from build123d import *

# Parameters (mm, degrees)
SKETCH1_W              = 121.666
SKETCH1_H              = 44.958
EXTRUDE1_DEPTH         = 152.4
SKETCH2_W              = 3.683
SKETCH2_H              = 43.292875233
EXTRUDE2_DEPTH         = 152.4
FILLET1_R              = 0.508
LPATTERN1_COUNT        = 23
LPATTERN1_PITCH        = 5.22224
FILLET1_OF_LPATTERN1_R = 0.508
SKETCH4_R              = 1.5875
EXTRUDE3_DEPTH         = 3.81
SKETCH5_R              = 1.5875
EXTRUDE4_DEPTH         = 3.81
SKETCH6_R              = 1.778
EXTRUDE5_DEPTH         = 3.81


with BuildPart() as part:
    # Sketch1 → Extrude1 (new body)
    with BuildSketch(Plane.XY):
        with Locations((60.833, 22.479)):
            Rectangle(SKETCH1_W, SKETCH1_H)
    extrude(amount=-EXTRUDE1_DEPTH)

    # Sketch2 → Extrude2 (cut)
    with BuildSketch(Plane.XY):
        with Locations((3.3655, 25.964437616)):
            Rectangle(SKETCH2_W, SKETCH2_H)
    extrude2 = extrude(amount=-EXTRUDE2_DEPTH, mode=Mode.SUBTRACT)

    # Fillet1
    fillet1_edges = [part.edges().sort_by_distance(p)[0] for p in [
        (1.524, 44.958, -76.2),
        (5.207, 44.958, -76.2),
    ]]
    fillet(fillet1_edges, radius=FILLET1_R)

    # LPattern1: Extrude2 ×23
    with Locations(*[(i * LPATTERN1_PITCH, 0, 0) for i in range(1, LPATTERN1_COUNT)]):
        add(extrude2, mode=Mode.SUBTRACT)

    # Fillet1 of LPattern1
    fillet1_of_lpattern1_edges = [part.edges().sort_by_distance(p)[0] for p in [
        (6.74624, 44.958, -76.2),
        (10.42924, 44.958, -76.2),
        (11.96848, 44.958, -76.2),
        (15.65148, 44.958, -76.2),
        (17.19072, 44.958, -76.2),
        (20.87372, 44.958, -76.2),
        (22.41296, 44.958, -76.2),
        (26.09596, 44.958, -76.2),
        (27.6352, 44.958, -76.2),
        (31.3182, 44.958, -76.2),
        (32.85744, 44.958, -76.2),
        (36.54044, 44.958, -76.2),
        (38.07968, 44.958, -76.2),
        (41.76268, 44.958, -76.2),
        (43.30192, 44.958, -76.2),
        (46.98492, 44.958, -76.2),
        (48.52416, 44.958, -76.2),
        (52.20716, 44.958, -76.2),
        (53.7464, 44.958, -76.2),
        (57.4294, 44.958, -76.2),
        (58.96864, 44.958, -76.2),
        (62.65164, 44.958, -76.2),
        (64.19088, 44.958, -76.2),
        (67.87388, 44.958, -76.2),
        (69.41312, 44.958, -76.2),
        (73.09612, 44.958, -76.2),
        (74.63536, 44.958, -76.2),
        (78.31836, 44.958, -76.2),
        (79.8576, 44.958, -76.2),
        (83.5406, 44.958, -76.2),
        (85.07984, 44.958, -76.2),
        (88.76284, 44.958, -76.2),
        (90.30208, 44.958, -76.2),
        (93.98508, 44.958, -76.2),
        (95.52432, 44.958, -76.2),
        (99.20732, 44.958, -76.2),
        (100.74656, 44.958, -76.2),
        (104.42956, 44.958, -76.2),
        (105.9688, 44.958, -76.2),
        (109.6518, 44.958, -76.2),
        (111.19104, 44.958, -76.2),
        (114.87404, 44.958, -76.2),
        (116.41328, 44.958, -76.2),
        (120.09628, 44.958, -76.2),
    ]]
    fillet(fillet1_of_lpattern1_edges, radius=FILLET1_OF_LPATTERN1_R)

    # Sketch4 → Extrude3 (cut)
    with BuildSketch(Plane.XZ):
        with Locations(Location((34.671, -43.18, 0), (0, 0, 270))):  # turned: the seam where the file's is
            Circle(SKETCH4_R)
        with Locations(Location((88.011, -109.22, 0), (0, 0, 270))):  # turned: the seam where the file's is
            Circle(SKETCH4_R)
    extrude(amount=-EXTRUDE3_DEPTH, mode=Mode.SUBTRACT)

    # Sketch5 → Extrude4 (cut)
    with BuildSketch(Plane.XZ):
        with Locations(Location((25.908, -43.18, 0), (0, 0, 270))):  # turned: the seam where the file's is
            Circle(SKETCH5_R)
        with Locations(Location((95.758, -109.22, 0), (0, 0, 270))):  # turned: the seam where the file's is
            Circle(SKETCH5_R)
    extrude(amount=-EXTRUDE4_DEPTH, mode=Mode.SUBTRACT)

    # Sketch6 → Extrude5 (cut)
    with BuildSketch(Plane.XZ):
        with Locations(Location((25.908, -13.081, 0), (0, 0, 270))):  # turned: the seam where the file's is
            Circle(SKETCH6_R)
        with Locations(Location((95.758, -13.081, 0), (0, 0, 270))):  # turned: the seam where the file's is
            Circle(SKETCH6_R)
        with Locations(Location((25.908, -63.9318, 0), (0, 0, 270))):  # turned: the seam where the file's is
            Circle(SKETCH6_R)
        with Locations(Location((95.758, -63.9318, 0), (0, 0, 270))):  # turned: the seam where the file's is
            Circle(SKETCH6_R)
        with Locations(Location((25.908, -140.081, 0), (0, 0, 270))):  # turned: the seam where the file's is
            Circle(SKETCH6_R)
        with Locations(Location((95.758, -140.081, 0), (0, 0, 270))):  # turned: the seam where the file's is
            Circle(SKETCH6_R)
    extrude(amount=-EXTRUDE5_DEPTH, mode=Mode.SUBTRACT)


solid = part.part
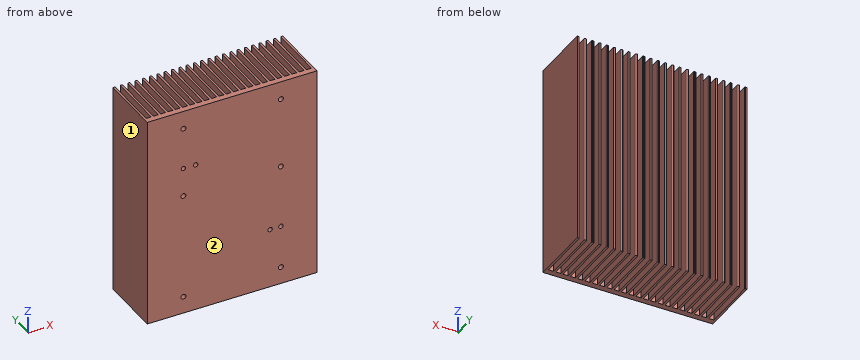
Geometry: final body of the model. Coordinates: model frame, mm. Face numbers are marked on the shaded views. Round coordinates to 2 decimals unless told otherwise and drop trailing zeros. Loops run counter-clockwise (first coordinate to the right, second up) from the corner with the lowest first, then second, coordinate; pieces in that order, holes last. Notation, with made-up numbers: (18, 29) - (40, 29) arc R28 cw to (40, 50) - close; hole circle Ø9 at (22, 53.5). An arc over 180 degrees is marked (long way). Write each question's results on one line, items separated by ' | '. Start each with the question number.
1) Line query: probe 1 along X at (y, z) = (2.4, -43.18); probe 2 along X at (y, z) = (1.65, -109.22); probe 3 along Y at (x, z) = (108, -51). Output: solid intervals per line, ascending. Write a range as [from, to].
2) Mould query, pull axis Y, two halves, no side actions, for the marked faces 1 and 2. Classes: released by +Y, released by -Y, zero draft, split by the parting line, or undercut.
3) Cut plane B-B on x = 66. Return loops of the section in (y, z).
4) First-contact query: P1, Ø3, axis at x = 69, z = -102, coming from the -Y side; P2, Ø1.8, axis at x = 19.5, z = -67, coming from the +Y side; P3, Ø1, axis at x = 26.5, z = -43.5, coming from the -Y side; P4, Ø4, axis at x = 81.5, z = -59, coming from the +Y side. Flat tips, straight axial feed; report the tip coordinate or a pass-through.
5) Cut plane A-A on y = 29.5. Count the separate pieces of the cut face and the enclosed holes in it, then the cut area to 3 significant figures.
Verdict:
1) probe 1: x = [0, 24.32], [27.5, 33.08], [36.26, 121.67] | probe 2: x = [0, 86.42], [89.6, 94.17], [97.35, 121.67] | probe 3: y = [0, 4.32]
2) face 1: zero draft | face 2: released by -Y
3) outline: (0, -152.4) - (4.32, -152.4) - (4.32, 0) - (0, 0) - close
4) P1: stops at y = 0 | P2: stops at y = 4.32 | P3: stops at y = 3.81 | P4: stops at y = 44.94
5) separate pieces: 24 | enclosed holes: 0 | area: 5,630 mm2
